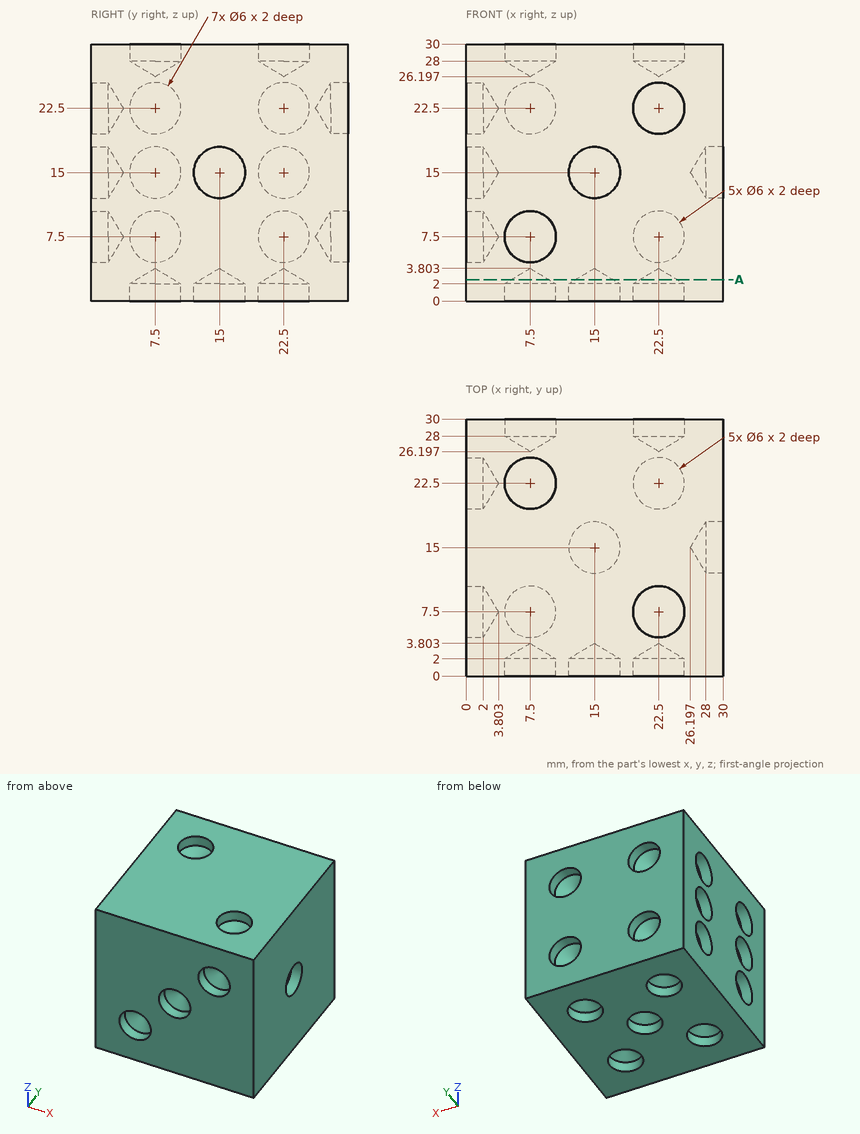
The drawing under review shows one solid part. Ordinate dimensions are in mm from its lowest x, y, z. Round coordinates to 2 decimals unless told otherwise and drop trailing zeros. Order: outer loops, then holes, each group sorted by start corner. A loop starts at its lowest first (then second) coordinate and runs counter-clockwise, first axis right, second up. Notation, with made-up numbers: (-4.75, 82.25) -> (25.25, 82.25) arc R18 cw to (25.25, 103.25) -> close; hole circle Ø2 at (82.25, -4.5). An arc over 180 degrees is marked (long way). Return JSON: item names as keys, results as strings.
1. Take a section at A-A (z = 2.5). Write out the cut boundary in (x, y) (1 decimal), then the cut area to 3 significant figures.
Answer block:
{"outline": "(0, 0) -> (30, 0) -> (30, 30) -> (0, 30) -> close; hole circle Ø4.3 at (7.5, 7.5); hole circle Ø4.3 at (7.5, 22.5); hole circle Ø4.3 at (15, 15); hole circle Ø4.3 at (22.5, 7.5); hole circle Ø4.3 at (22.5, 22.5)", "area": "826 mm²"}
2. For L1, parallel to Y at x = 0.6, z = 22.5; L2, parallel to Z at x = 0.9, y = 7.5; L3, parallel to X at y = 15, z = 0.55, list the stretches that pass through material, from the lowest coordinate up. Write a range as [from, to].
Answer block:
{"L1": "y = [0, 4.5], [10.5, 19.5], [25.5, 30]", "L2": "z = [0, 4.5], [10.5, 12], [18, 19.5], [25.5, 30]", "L3": "x = [0, 12], [18, 30]"}
3. Insertion check: P1, Ø5.5, axis at x = 22.5, z = 22.5, coming from the -Y side; P2, Ø3.5, axis at x = 7.5, z = 7.5, coming from the -Y side; P3, Ø5, axis at x = 22.5, z = 22.5, coming from the +Y side. Each pin has a flat end and moves straight along its axis. Give the tip position at first contact, or say it passes through.
Answer block:
{"P1": "stops at y = 2.15", "P2": "stops at y = 2.75", "P3": "stops at y = 27.7"}
